Check sheet for the modelled part. Datum: model origin and axes. Units: mm. A direction names the side the tool comes from. Give positions to 0.01 mm unless a question says otherwise; leave off trailing zeros. Order: outer loops, then holes, each group sorted by start corner. A loop starts at its lowest first (then second) coordinate and runs counter-clockwise, first axis right, second up. Notation, with made-up numbers: (47, -12.75) -> (99, -12.75) arc R11 ccw to (99, -1.75) -> close; hole circle Ø1 at (46.25, -3). An arc over 180 degrees is marked (long way). Answer in a Markdown table with one row per item. Add a question column.
(1) Thickness scan on L1, parallel to X at y = -39, z = 0.95; L2, parallel to Y at x = 24.5, z = 2.3; L3, parallel to Y at x = -24.5, z = 1.3. Record the ranges inside material, lowest first. Write a range as [from, to].
(2) Go/stop test with flat-tipped pins: pin 1 (4.5 mm diameter, centred on x = -24.5, y = 39, fed in from +Z); pin 2 (7.5 mm diameter, centred on x = -24.5, y = 39, fed in from +Z); pin 3 (4.5 mm diameter, centred on x = 24, y = 40.5, fed in from +Z). Record where each tip stops, or that it passes through.
(3) Cross-section at C-C (z = 3.85). Record the cut outline in (x, y), then the cut area to 3 significant figures.
(4) Release check for a two-part mould opening along X. For faces 3 (the face through (-31.43, 0.65, 4.4)), 4 (the face through (-26, -38, 2)), 5 (the face through (32, -1, 1)), 6 (the face through (0.45, 45.93, 4.4)) record: released by +X, released by -X, zero draft, split by the parting line, or undercut.
(5) Cross-section at B-B (x = -24.5). Record the cut outline in (y, z).
(6) Set-up check for faces 1 (the face through (-26.801, 37.235, 2.507)), 2 (the face through (-23.284, -40.115, 0.986)): record each of +Z, -Z, +X, -X, +Y, -Y from which the full face is reachable in a straight line by a thin tool's end or side.
(7) Cross-section at A-A (y = -39). Record the cut outline in (x, z).
```python
from build123d import *

# Parameters (mm, degrees)
SKIZZE1_W                       = 64
SKIZZE1_H                       = 93
SKIZZE1_R                       = 1.65
AUFSATZ_LINEAR_AUSTRAGEN2_DEPTH = 5
SKIZZE2_R                       = 2.9
SCHNITT_LINEAR_AUSTRAGEN1_DEPTH = 3
VERRUNDUNG1_R                   = 2


with BuildPart() as part:
    # Skizze1 → Aufsatz-Linear austragen2 (new body)
    with BuildSketch(Plane.XY):
        Rectangle(SKIZZE1_W, SKIZZE1_H)
        with Locations((-24.5, 39)):
            Circle(SKIZZE1_R, mode=Mode.SUBTRACT)
        with Locations(Location((24.5, 39, 0), (0, 0, 180))):
            Circle(SKIZZE1_R, mode=Mode.SUBTRACT)
        with Locations((24.5, -39)):
            Circle(SKIZZE1_R, mode=Mode.SUBTRACT)
        with Locations(Location((-24.5, -39, 0), (0, 0, 180))):
            Circle(SKIZZE1_R, mode=Mode.SUBTRACT)
    extrude(amount=AUFSATZ_LINEAR_AUSTRAGEN2_DEPTH)

    # Skizze2 → Schnitt-Linear austragen1 (cut)
    with BuildSketch(Plane.XY.offset(5)):
        with Locations((-24.5, 39)):
            Circle(SKIZZE2_R)
        with Locations(Location((24.5, 39, 0), (0, 0, 180))):
            Circle(SKIZZE2_R)
        with Locations((24.5, -39)):
            Circle(SKIZZE2_R)
        with Locations(Location((-24.5, -39, 0), (0, 0, 180))):
            Circle(SKIZZE2_R)
    extrude(amount=-SCHNITT_LINEAR_AUSTRAGEN1_DEPTH, mode=Mode.SUBTRACT)

    # Verrundung1
    verrundung1_edges = [part.edges().sort_by_distance(p)[0] for p in [
        (-32, 0, 5),
        (0, -46.5, 5),
        (-21.6, -39, 5),
        (21.6, -39, 5),
        (27.4, 39, 5),
        (-27.4, 39, 5),
        (32, 0, 5),
        (0, 46.5, 5),
    ]]
    fillet(verrundung1_edges, radius=VERRUNDUNG1_R)


solid = part.part
```
Answer below:
| question | item | result |
|---|---|---|
| 1 | L1 | x = [-32, -26.15], [-22.85, 22.85], [26.15, 32] |
| 1 | L2 | y = [-46.5, -41.9], [-36.1, 36.1], [41.9, 46.5] |
| 1 | L3 | y = [-46.5, -40.65], [-37.35, 37.35], [40.65, 46.5] |
| 2 | pin 1 | stops at z = 2 |
| 2 | pin 2 | stops at z = 4.64 |
| 2 | pin 3 | stops at z = 4.69 |
| 3 | outline | (-31.81, -46.31) -> (31.81, -46.31) -> (31.81, 46.31) -> (-31.81, 46.31) -> close; hole circle Ø6.18 at (-24.5, -39); hole circle Ø6.18 at (-24.5, 39); hole circle Ø6.18 at (24.5, -39); hole circle Ø6.18 at (24.5, 39) |
| 3 | area | 5,770 mm² |
| 4 | face 3 | released by -X |
| 4 | face 4 | undercut |
| 4 | face 5 | released by +X |
| 4 | face 6 | zero draft |
| 5 | outline | (-46.5, 0) -> (-40.65, 0) -> (-40.65, 2) -> (-41.9, 2) -> (-41.9, 3) arc R2 ccw to (-43.9, 5) -> (-44.5, 5) arc R2 ccw to (-46.5, 3) -> close; (-37.35, 0) -> (37.35, 0) -> (37.35, 2) -> (36.1, 2) -> (36.1, 3) arc R2 ccw to (34.1, 5) -> (-34.1, 5) arc R2 ccw to (-36.1, 3) -> (-36.1, 2) -> (-37.35, 2) -> close; (40.65, 0) -> (46.5, 0) -> (46.5, 3) arc R2 ccw to (44.5, 5) -> (43.9, 5) arc R2 ccw to (41.9, 3) -> (41.9, 2) -> (40.65, 2) -> close |
| 6 | face 1 | +Z |
| 6 | face 2 | +Z, -Z |
| 7 | outline | (-32, 0) -> (-26.15, 0) -> (-26.15, 2) -> (-27.4, 2) -> (-27.4, 3) arc R2 ccw to (-29.4, 5) -> (-30, 5) arc R2 ccw to (-32, 3) -> close; (-22.85, 0) -> (22.85, 0) -> (22.85, 2) -> (21.6, 2) -> (21.6, 3) arc R2 ccw to (19.6, 5) -> (-19.6, 5) arc R2 ccw to (-21.6, 3) -> (-21.6, 2) -> (-22.85, 2) -> close; (26.15, 0) -> (32, 0) -> (32, 3) arc R2 ccw to (30, 5) -> (29.4, 5) arc R2 ccw to (27.4, 3) -> (27.4, 2) -> (26.15, 2) -> close |
